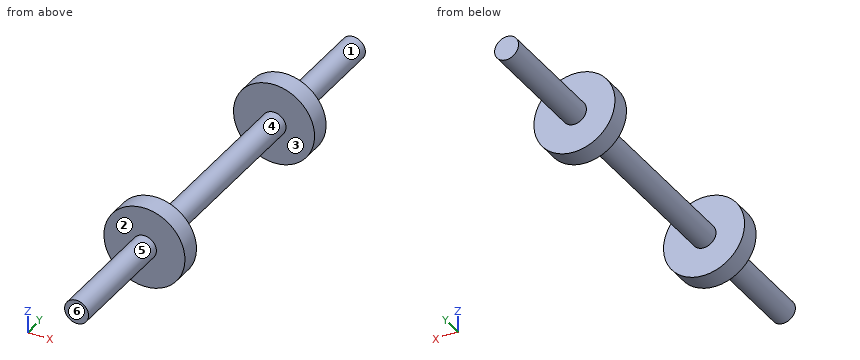
from build123d import *

# Parameters (mm, degrees)
SKETCH1_R           = 7.5
BOSS_EXTRUDE1_DEPTH = 304.8
SKETCH2_W           = 25.4
SKETCH2_H           = 12.7


with BuildPart() as part:
    # Sketch1 → Boss-Extrude1 (new body)
    with BuildSketch(Plane(origin=(0, 0, 0), x_dir=(1, 0, 0), z_dir=(0, 1, 0))):
        with Locations(Location((0, 0, 0), (0, 0, 90))):
            Circle(SKETCH1_R)
    extrude(amount=BOSS_EXTRUDE1_DEPTH)

    # Sketch2 → Revolve1 (revolve)
    with BuildSketch(Plane.XY, mode=Mode.PRIVATE) as revolve1_sk:
        with Locations((12.7, 223.75)):
            Rectangle(SKETCH2_W, SKETCH2_H)
        with Locations((12.7, 81.05)):
            Rectangle(SKETCH2_W, SKETCH2_H)
    revolve(revolve1_sk.sketch.rotate(Axis((0, 217.4, 0), (0, 1, 0)), 90), axis=Axis((0, 217.4, 0), (0, 1, 0)))


solid = part.part
The listing builds one solid part. Answer for the finished solid, in the listing's coordinates (mm). Face numbers are marked on the shaded views. A direction names the side the tool comes from. Give positions to 0.01 mm unless a question says otherwise; leave off trailing zeros. Write each loop counter-clockwise with the first axis right and the second up, starting at its lowest first coordinate (ties: lowest second). Pieces come first, ordered by that corner, then holes. Notation, with made-up numbers: (41, -36) - (76, -36) arc R19 cw to (76, -7) - close; hole circle Ø9 at (40.25, 9). An arc over 180 degrees is marked (long way). Use a Markdown table: item, result.
1. Section A-A on x = 19.5 is taken. Write down the section's boundary in (y, z).
Values follow:
| item | result |
|---|---|
| outline | (74.7, -16.28) - (87.4, -16.28) - (87.4, 16.28) - (74.7, 16.28) - close; (217.4, -16.28) - (230.1, -16.28) - (230.1, 16.28) - (217.4, 16.28) - close |
2. Find the intervals of material crossed by probe 1 along Y at (x, z) = (-1, -15.5); probe 2 along Z at (x, y) = (-16, 221.5); probe 3 along Z at (x, y) = (4, 50.5), in increasing order. Write a range as from..to.
Values follow:
| item | result |
|---|---|
| probe 1 | y = 74.7..87.4, 217.4..230.1 |
| probe 2 | z = -19.73..19.73 |
| probe 3 | z = -6.34..6.34 |
3. Each of these flat-tipped pins is pushed along its axis until it touches: P1, Ø3, axis at x = 3, y = 45.5, coming from the +Z side; P2, Ø10, axis at x = 10, y = 248, coming from the -Z side; P3, Ø8, axis at x = -5.5, z = -19, coming from the +Y side; P4, Ø12, axis at y = 149.5, z = 16, coming from the -X side. Where does it stop, or does it pass through?
Values follow:
| item | result |
|---|---|
| P1 | stops at z = 7.35 |
| P2 | stops at z = -5.59 |
| P3 | stops at y = 230.1 |
| P4 | passes through |
4. Section C-C on x = 0 is taken. Write down the section's boundary in (y, z), plus the area to 3 significant figures.
Values follow:
| item | result |
|---|---|
| outline | (0, -7.5) - (74.7, -7.5) - (74.7, -25.4) - (87.4, -25.4) - (87.4, -7.5) - (217.4, -7.5) - (217.4, -25.4) - (230.1, -25.4) - (230.1, -7.5) - (304.8, -7.5) - (304.8, 7.5) - (230.1, 7.5) - (230.1, 25.4) - (217.4, 25.4) - (217.4, 7.5) - (87.4, 7.5) - (87.4, 25.4) - (74.7, 25.4) - (74.7, 7.5) - (0, 7.5) - close |
| area | 5,480 mm² |
5. Section B-B on z = 12 is taken. Write down the section's boundary in (x, y).
Values follow:
| item | result |
|---|---|
| outline | (-22.39, 74.7) - (22.39, 74.7) - (22.39, 87.4) - (-22.39, 87.4) - close; (-22.39, 217.4) - (22.39, 217.4) - (22.39, 230.1) - (-22.39, 230.1) - close |
6. A tool of negligible diameter and unlimited length cuts with its end or side. For the marked faces 1, 2 and 3, from which of +Z, -Z, +X, -X, +Y, -Y can it reach the whole face along a straight path? Write none if from no direction.
Values follow:
| item | result |
|---|---|
| face 1 | +Y |
| face 2 | -Y |
| face 3 | none |
7. Section D-D on z = 0 is taken. Write down the section's boundary in (x, y), plus the area to 3 significant figures.
Values follow:
| item | result |
|---|---|
| outline | (-25.4, 74.7) - (-7.5, 74.7) - (-7.5, 0) - (7.5, 0) - (7.5, 74.7) - (25.4, 74.7) - (25.4, 87.4) - (7.5, 87.4) - (7.5, 217.4) - (25.4, 217.4) - (25.4, 230.1) - (7.5, 230.1) - (7.5, 304.8) - (-7.5, 304.8) - (-7.5, 230.1) - (-25.4, 230.1) - (-25.4, 217.4) - (-7.5, 217.4) - (-7.5, 87.4) - (-25.4, 87.4) - close |
| area | 5,480 mm² |
8. For a pull along Y with two mould halves and no side action, classify the marked faces 4, 5 and 6 as released by +Y, released by -Y, zero draft, split by the parting line, or undercut.
Values follow:
| item | result |
|---|---|
| face 4 | undercut |
| face 5 | zero draft |
| face 6 | released by -Y |
